Can you work these out from the model? Positions are in its coordinate system, mm. Round coordinates to 2 decimals unless told otherwise and drop trailing zeros. Write each loop counter-clockwise with the first axis right and the second up, starting at its lowest first coordinate (ties: lowest second). Pieces come first, ordered by that corner, then holes. Notation, with made-up numbers: M -35.5,31.25 L -1.5,31.25 A26 ccw -1.5,47.25 Z; hole C 0,43.25 d2. An arc over 180 degrees is marked long. Answer in a Markdown table with one row per item. Add a question column.
(1) If we mould it in two halves opening along X, with no side actions, what happens to faces 1 (the face through (7, 1, -3.5)), 2 (the face through (-3.5, 1.5, 0.1)), 3 (the face through (8.3, 1.5, 1.5))? For each: released by +X, released by -X, zero draft, split by the parting line, or undercut.
(2) If I drill on probe 1 along X at (y, z) = (1.2, 0); probe 2 along Z at (x, y) = (14, 0.7); probe 3 along Z at (x, y) = (0, 1.8), over which ranges is the centre line in solid material (lowest first)?
(3) Suppose I cut it at A-A, the plane y = 2.55. Write out the boundary of the cut face in (x, z).
(4) Suppose I cut it at D-D, the plane x = 13. Write out the boundary of the cut face in (y, z).
(5) Suppose I cut it at B-B, the plane z = 0. Write out the boundary of the cut face in (x, y), then the cut area to 3 significant figures.
(6) Suppose I cut it at C-C, the plane x = -0.75. Write out the boundary of the cut face in (y, z).
from build123d import *

# Parameters (mm, degrees)
SKETCH1_R           = 0.75
SKETCH1_R_2         = 1
BOSS_EXTRUDE1_DEPTH = 3
CUT_EXTRUDE1_DEPTH  = 10


with BuildPart() as part:
    # Sketch1 → Boss-Extrude1 (new body)
    with BuildSketch(Plane(origin=(0, 0, 0), x_dir=(1, 0, 0), z_dir=(0, 1, 0))):
        with BuildLine():
            Line((0, 3.5), (14, 3.5))
            ThreePointArc((14, 3.5), (17.5, 0), (14, -3.5))
            Line((14, -3.5), (0, -3.5))
            ThreePointArc((0, -3.5), (-3.5, 0), (0, 3.5))
        make_face()
        with Locations((14, 0)):
            Circle(SKETCH1_R, mode=Mode.SUBTRACT)
        Circle(SKETCH1_R_2, mode=Mode.SUBTRACT)
    extrude(amount=BOSS_EXTRUDE1_DEPTH)

    # Sketch2 → Cut-Extrude1 (cut)
    with BuildSketch(Plane(origin=(0, 3, 0), x_dir=(1, 0, 0), z_dir=(0, 1, 0))):
        with BuildLine():
            Line((2.916994756, -3.5), (13.5, -3.5))
            ThreePointArc((13.5, -3.5), (8.208497378, -1.5), (2.916994756, -3.5))
        make_face()
    extrude(amount=-CUT_EXTRUDE1_DEPTH, mode=Mode.SUBTRACT)


solid = part.part
Calculated:
| question | item | result |
|---|---|---|
| 1 | face 1 | zero draft |
| 1 | face 2 | released by -X |
| 1 | face 3 | undercut |
| 2 | probe 1 | -3.5 to -1, 1 to 13.25, 14.75 to 17.5 |
| 2 | probe 2 | -3.5 to -0.75, 0.75 to 3.5 |
| 2 | probe 3 | -3.5 to -1, 1 to 3.5 |
| 3 | outline | M 0,-3.5 L 14,-3.5 A3.5 ccw 14,3.5 L 13.5,3.5 A8 cw 2.92,3.5 L 0,3.5 A3.5 ccw Z; hole C 0,0 d2; hole C 14,0 d1.5 |
| 4 | outline | M 0,-3.5 L 3,-3.5 L 3,3.09 L 0,3.09 Z |
| 5 | outline | M -3.5,0 L -1,0 L -1,3 L -3.5,3 Z; M 1,0 L 13.25,0 L 13.25,3 L 1,3 Z; M 14.75,0 L 17.5,0 L 17.5,3 L 14.75,3 Z |
| 5 | area | 52.5 mm² |
| 6 | outline | M 0,-3.42 L 3,-3.42 L 3,-0.66 L 0,-0.66 Z; M 0,0.66 L 3,0.66 L 3,3.42 L 0,3.42 Z |
